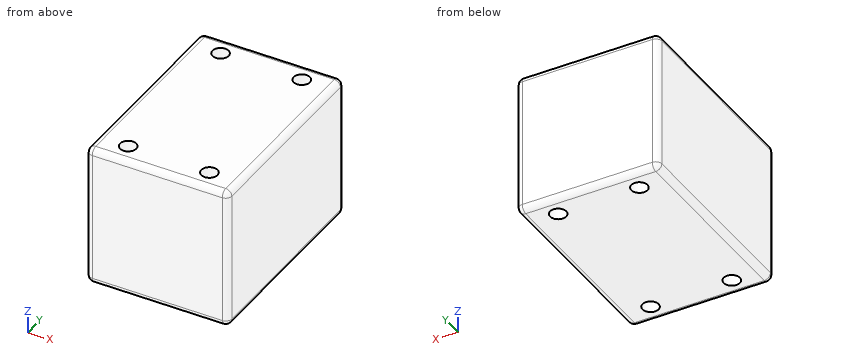
from build123d import *

# Parameters (mm, degrees)
SKETCH1_W           = 70
SKETCH1_H           = 100
BOSS_EXTRUDE1_DEPTH = 70
SKETCH2_R           = 4
CUT_EXTRUDE1_DEPTH  = 93.870878105
FILLET1_R           = 3


with BuildPart() as part:
    # Sketch1 → Boss-Extrude1 (new body)
    with BuildSketch(Plane.XY):
        Rectangle(SKETCH1_W, SKETCH1_H)
    extrude(amount=BOSS_EXTRUDE1_DEPTH)

    # Sketch2 → Cut-Extrude1 (cut, through all)
    with BuildSketch(Plane.XY.offset(70)):
        with Locations((-20, 40)):
            Circle(SKETCH2_R)
        with Locations(Location((-20, -40, 0), (0, 0, 180))):
            Circle(SKETCH2_R)
        with Locations((20, -40)):
            Circle(SKETCH2_R)
        with Locations(Location((20, 40, 0), (0, 0, 180))):
            Circle(SKETCH2_R)
    extrude(amount=-CUT_EXTRUDE1_DEPTH, mode=Mode.SUBTRACT)

    # Fillet1
    fillet1_edges = [part.edges().sort_by_distance(p)[0] for p in [
        (-35, 0, 70),
        (0, -50, 70),
        (35, 0, 70),
        (0, -50, 0),
        (-35, 0, 0),
        (0, 50, 0),
        (35, 0, 0),
        (0, 50, 70),
        (35, -50, 35),
        (-35, -50, 35),
        (-35, 50, 35),
        (35, 50, 35),
    ]]
    fillet(fillet1_edges, radius=FILLET1_R)


solid = part.part
Verification items for the finished model (mm, model axes). Coordinates: 2 decimals unless noted, no trailing zeros. Order: outer loops, then holes, each group sorted by start corner. A loop starts at its lowest first (then second) coordinate and runs counter-clockwise, first axis right, second up. Notation, with made-up numbers: M 62,-37 L 119,-37 A34 cw 119,-7 Z; hole C 35,-6.75 d1. An arc over 180 degrees is marked long. Write each question's results on one line, items separated by ' | '.
1) Section check C-C on z = 59. Record the cut outline in (x, y).
Solved:
outline: M -35,-47 A3 ccw -32,-50 L 32,-50 A3 ccw 35,-47 L 35,47 A3 ccw 32,50 L -32,50 A3 ccw -35,47 Z; hole C -20,-40 d8; hole C -20,40 d8; hole C 20,-40 d8; hole C 20,40 d8
2) Section check A-A on y = 40. Record the cut outline in (x, z), plus the area to 3 significant figures.
Solved:
outline: M -35,3 A3 ccw -32,0 L -24,0 L -24,70 L -32,70 A3 ccw -35,67 Z; M -16,0 L 16,0 L 16,70 L -16,70 Z; M 24,0 L 32,0 A3 ccw 35,3 L 35,67 A3 ccw 32,70 L 24,70 Z | area: 3,770 mm²
3) Scan lines: line 1 along Y through (x, z) = (20, 28); line 2 along Y through (x, z) = (18, 34.5); line 3 along X through (y, z) = (41.5, 8). Record each from-to range of solid material in increasing order. Write a range as [from, to].
Solved:
line 1: y = [-50, -44], [-36, 36], [44, 50] | line 2: y = [-50, -43.46], [-36.54, 36.54], [43.46, 50] | line 3: x = [-35, -23.71], [-16.29, 16.29], [23.71, 35]
4) Section check B-B on x = 20. Record the cut outline in (y, z), plus the area to 3 significant figures.
Solved:
outline: M -50,3 A3 ccw -47,0 L -44,0 L -44,70 L -47,70 A3 ccw -50,67 Z; M -36,0 L 36,0 L 36,70 L -36,70 Z; M 44,0 L 47,0 A3 ccw 50,3 L 50,67 A3 ccw 47,70 L 44,70 Z | area: 5,870 mm²
